```python
from build123d import *

# Parameters (mm, degrees)
F0_R     = 10
F0_R_2   = 2.85
F0_R_3   = 1.6
F1_DEPTH = 15
F2_SIZE  = 4
F3_DEPTH = 2.04


with BuildPart() as f1:
    # F0 (on Top) → F1 (new body)
    with BuildSketch(Plane.XY):
        Circle(F0_R)
        Circle(F0_R_2, mode=Mode.SUBTRACT)
        Circle(F0_R_2)
        Circle(F0_R_3, mode=Mode.SUBTRACT)
    extrude(amount=F1_DEPTH)

    # F2
    f2_edges = [f1.edges().sort_by_distance(p)[0] for p in [
        (10, 0, 7.5),
        (-10, 0, 0),
        (-10, 0, 15),
    ]]
    chamfer(f2_edges, length=F2_SIZE)

    # F0 (on Top) → F3 (cut)
    with BuildSketch(Plane.XY):
        Circle(F0_R_2)
        Circle(F0_R_3, mode=Mode.SUBTRACT)
    extrude(amount=F3_DEPTH, mode=Mode.SUBTRACT)


solid = f1.part
```
Build history of the part. All positions in model axes, mm. A direction names the side the tool comes from. Give positions to 0.01 mm unless a question says otherwise; leave off trailing zeros. Order: outer loops, then holes, each group sorted by start corner. A loop starts at its lowest first (then second) coordinate and runs counter-clockwise, first axis right, second up. Notation, with made-up numbers: M -10,-33.75 L 34,-33.75 A34 ccw 34,1.25 Z; hole C 56.5,81 d7. An arc over 180 degrees is marked long. Write item = value, one per line. Start each with the question number.
(1) Slice it at C-C on z = 7.75. Write the cut outline in (x, y), plus the area to 3 significant figures.
(2) Slice it at D-D on z = 14. Write the cut outline in (x, y).
(3) Which spindle directions (+Z, -Z, +X, -X, +Y, -Y) get a long thin tool onto all of the face, cutting with end or side? Do faces 1 (the cylindrical face through (-1.27, -0.97, 8.43)), 2 (the flat face through (0, -2, 2.04)). Say none if no direction does.
(4) Two-plate mould, pull along X, no slides. Class faces 3 (the cylindrical face through (-2.17, -9.76, 7.45)), 4 (the cylindrical face through (-2.262, -1.734, 1.006)), 5 (the flat face through (1.25, -1.25, 15)): released by +X, released by -X, zero draft, split by the parting line, or undercut.
(5) Pin check, flat tips, straight feed: pin 1 Ø3 at (x, y) = (-1, 2) entering from -Z; pin 2 Ø6 at (x, z) = (6, 7.5) entering from -Y; pin 3 Ø3 at (x, z) = (2.5, 11) entering from -Y; pin 4 Ø3 at (x, y) = (6.5, 5.5) entering from -Z. Stop position of each tip, or through.
(6) Slice it at A-A on x = 0. Write the cut outline in (y, z).
(7) Probe L1, parallel to Y at x = 0, z = 9.25; L2, parallel to Z at x = 0, y = 2.5; L3, parallel to Y at x = 0.75, z = 13.5. List the from-to ranges inside material, lowest first. Write a range as [from, to].
Responses:
q1.outline = C 0,0 d20; hole C 0,0 d3.2
q1.area = 306 mm2
q2.outline = C 0,0 d14; hole C 0,0 d3.2
q3.face_1 = +Z, -Z
q3.face_2 = -Z
q4.face_3 = split by the parting line
q4.face_4 = undercut
q4.face_5 = zero draft
q5.pin_1 = 0
q5.pin_2 = -9.54
q5.pin_3 = -9.95
q5.pin_4 = 1.01
q6.outline = M -10,4 L -6,0 L -2.85,0 L -2.85,2.04 L -1.6,2.04 L -1.6,15 L -6,15 L -10,11 Z; M 1.6,2.04 L 2.85,2.04 L 2.85,0 L 6,0 L 10,4 L 10,11 L 6,15 L 1.6,15 Z
q7.L1 = [-10, -1.6], [1.6, 10]
q7.L2 = [2.04, 15]
q7.L3 = [-7.46, -1.41], [1.41, 7.46]
